Autodesk Inventor part; units mm, degrees
ref_plane "YZ Plane" through (0, 0, 0) normal (1, 0, 0) x (0, 1, 0)
ref_plane "XZ Plane" through (0, 0, 0) normal (0, 1, 0) x (-1, 0, 0)
ref_plane "XY Plane" through (0, 0, 0) normal (0, 0, 1) x (1, 0, 0)
sketch "Sketch1" plane through (0, 0, 0) normal (0, 1, 0) x (-1, 0, 0)
  line L0 (23.1483, 102.1323) -> (7.9083, 102.1323)
  line L1 (7.9083, 102.1323) -> (7.9083, -75.6677)
  line L2 (7.9083, -75.6677) -> (23.1483, -75.6677)
  line L3 (23.1483, -75.6677) -> (23.1483, 102.1323)
  point P0 (0, 0)
  dimension "d0" = 177.8
  dimension "d1" = 15.24
extrude "Extrusion1" add sketch "Sketch1" along normal blind 7.62
sketch "Sketch2" plane through (0, 7.62, 0) normal (0, 1, 0) x (1, 0, 0)
  line L0 (-23.1483, 75.6677) -> (-23.1483, -102.1323)
  line L1 (-7.9083, 75.6677) -> (-23.1483, 75.6677)
  line L2 (-23.1483, -102.1323) -> (-7.9083, -102.1323)
  point P0 (0, 0)
  point P1 (-15.5283, -64.0323)
  point P2 (-15.5283, 37.5677)
  dimension "d4" = 0
  dimension "d5" = 101.6
  dimension "d6" = 7.62
  dimension "d7" = 38.1
  dimension "d8" = 38.1
hole "Hole1" at (-15.5283, 7.62, 64.0323) at (-15.5283, 7.62, -37.5677) direction (0, -1, 0) diameter 2.794 end through all
sketch "Sketch3" plane through (0, 7.62, 0) normal (0, 1, 0) x (1, 0, 0)
  circle A0 centre (-15.5283, -64.0323) radius 1.397
  circle A1 centre (-15.5283, 37.5677) radius 1.397
  circle A2 centre (-15.5283, -64.0323) radius 3.175
  circle A3 centre (-15.5283, 37.5677) radius 3.175
  point P0 (0, 0)
  dimension "d16" = 6.35
  dimension "d17" = 6.35
extrude "Extrusion2" cut sketch "Sketch3" against normal blind 3.048
sketch "Sketch4" plane through (0, 7.62, 0) normal (0, 1, 0) x (1, 0, 0)
  line L0 (-7.9083, -102.1323) -> (-7.9083, 75.6677)
  line L1 (-23.1483, -102.1323) -> (-7.9083, -102.1323)
  line L2 (-7.9083, 75.6677) -> (-23.1483, 75.6677)
  point P0 (0, 0)
  point P1 (-15.5283, -91.9723)
  point P2 (-15.5283, 65.5077)
  dimension "d20" = 0
  dimension "d21" = 7.62
  dimension "d22" = 10.16
  dimension "d23" = 10.16
hole "Hole2" at (-15.5283, 7.62, 91.9723) at (-15.5283, 7.62, -65.5077) direction (0, -1, 0) diameter 4.826 end through all
properties part number "RioConnectors"
Read the model definition and answer for the solid it produces. Units are mm, in the model's axes. A direction names the side the tool comes from. Round coordinates to 2 decimals unless told otherwise and drop trailing zeros. Write each loop counter-clockwise with the first axis right and the second up, starting at its lowest first coordinate (ties: lowest second). Pieces come first, ordered by that corner, then holes.
1. Determine the mould class of faces 3 (the face through (-23.148, 4, 12)), 4 (the face through (-15, 7.62, 14)), 5 (the face through (-16.253, 3.757, 94.274)) for opening direction X: pulls with the +X half, pulls with the -X half, needs draft (parallel to the pull), parting line crosses it, or undercut.
2. Straight lines are drawn through the part: L1, parallel to Z at x = -15.25, y = 6.5; L2, parallel to Z at x = -17.5, y = 3.75; L3, parallel to Z at x = -17, y = 1.75. For each, find the intervals that lie inside material, in ascending order.
3. Given pin 1 Ø1.9 at (x, z) = (-17, 62.5) entering from +Y; pin 2 Ø2.5 at (x, z) = (-15.53, -37.57) entering from -Y, each flat-ended and moving along its own axis, determine where each tip first touches the part or whether it passes through.
4. Which of the six approach directions +Z, -Z, +X, -X, +Y, -Y give full straight-line access (tool end or side, diameter ignored) to faces 1 (the face through (-16.47, 2.25, 63)), 2 (the face through (-14, 4.572, 65))?
5. The part is cut by section A-A, the plane y = 2.75. Determine the outline of the cut face in (x, z), then the cut area to 3 significant figures.
Values:
1. face 3: pulls with the -X half
1. face 4: needs draft
1. face 5: undercut
2. L1: z = -75.67 to -67.9, -63.11 to -40.73, -34.4 to 60.87, 67.2 to 89.58, 94.37 to 102.13
2. L2: z = -75.67 to -66.9, -64.12 to 90.58, 93.36 to 102.13
2. L3: z = -75.67 to -67.42, -63.6 to 90.06, 93.88 to 102.13
3. pin 1: stops at y = 4.57
3. pin 2: passes through
4. face 1: +Y, -Y
4. face 2: +Y
5. outline: (-23.15, -75.67) - (-7.91, -75.67) - (-7.91, 102.13) - (-23.15, 102.13) - close; hole circle Ø4.83 at (-15.53, -65.51); hole circle Ø4.83 at (-15.53, 91.97); hole circle Ø2.79 at (-15.53, -37.57); hole circle Ø2.79 at (-15.53, 64.03)
5. area: 2,660 mm2
